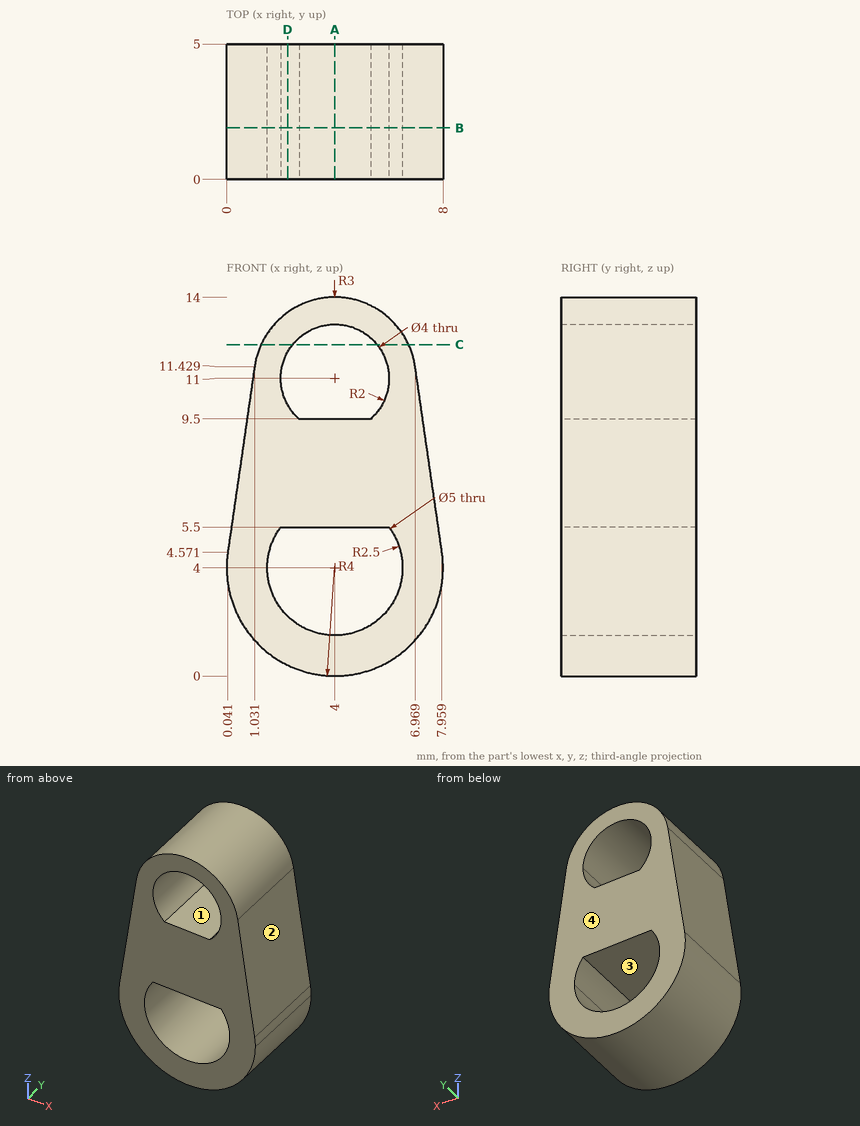
Can you work these out from the drawing? Everything is in mm from the part's minimum corner. Round coordinates to 2 decimals unless told otherwise and drop trailing zeros. Order: outer loops, then holes, each group sorted by start corner. A loop starts at its lowest first (then second) coordinate and runs counter-clockwise, first axis right, second up. Notation, with made-up numbers: M 51,17.5 L 74,17.5 A6 ccw 74,27.5 Z; hole C 41,-5 d10. An arc over 180 degrees is marked long. One line per question, with ' | ' between items.
1) I want a section at A-A, the plane x = 4. Write out the boundary of the cut face in (y, z), then the cut area to 3 significant figures.
Working result:
outline: M 0,0 L 5,0 L 5,1.5 L 0,1.5 Z; M 0,5.5 L 5,5.5 L 5,9.5 L 0,9.5 Z; M 0,13 L 5,13 L 5,14 L 0,14 Z | area: 32.5 mm²
2) I want a section at B-B, the plane y = 1.9. Write out the boundary of the cut face in (x, z).
Working result:
outline: M 0.04,4.57 A4 ccw long 8,4 A4 ccw 7.96,4.57 L 6.97,11.43 A3 ccw 1.03,11.43 Z; hole M 2,5.5 A2.5 ccw long 6.5,4 A2.5 ccw 6,5.5 Z; hole M 2.68,9.5 L 5.32,9.5 A2 ccw 6,11 A2 ccw long Z
3) For pin 1 Ø1 at (y, z) = (3.5, 5.5) entering from -X; pin 2 Ø2 at (x, y) = (2.5, 0.5) entering from +Z, each with a flat end and sliding along its axis, tell me the tip position at first contact or that it passes through.
Working result:
pin 1: x = 0.1 | pin 2: z = 13.96
4) If we mould it in two halves opening along Z, with no side actions, what happens to the marked faces 1, 2, 3 and 4? For each: +Z half, -Z half, draft (parallel to the pull), parting line (faces both ways), or undercut.
Working result:
face 1: undercut | face 2: +Z half | face 3: undercut | face 4: draft
5) I want a section at D-D, the plane x = 2.25. Write out the boundary of the cut face in (y, z) (1 decimal).
Working result:
outline: M 0,0.4 L 5,0.4 L 5,2.2 L 0,2.2 Z; M 0,5.5 L 5,5.5 L 5,10 L 0,10 Z; M 0,12 L 5,12 L 5,13.4 L 0,13.4 Z
6) I want a section at C-C, the plane z = 12.25. Write out the boundary of the cut face in (x, y).
Working result:
outline: M 1.27,0 L 2.44,0 L 2.44,5 L 1.27,5 Z; M 5.56,0 L 6.73,0 L 6.73,5 L 5.56,5 Z
7) I need wall thicknesses on line 1 along Z through (x, y) = (4, 3.35); line 2 along Z through (x, y) = (2.75, 0.95) (1 decimal); line 3 along X through (y, z) = (0.85, 4). Which ranges of each line are inside material? Lowest first, please.
Working result:
line 1: 0 to 1.5, 5.5 to 9.5, 13 to 14 | line 2: 0.2 to 1.8, 5.5 to 9.5, 12.6 to 13.7 | line 3: 0 to 1.5, 6.5 to 8
